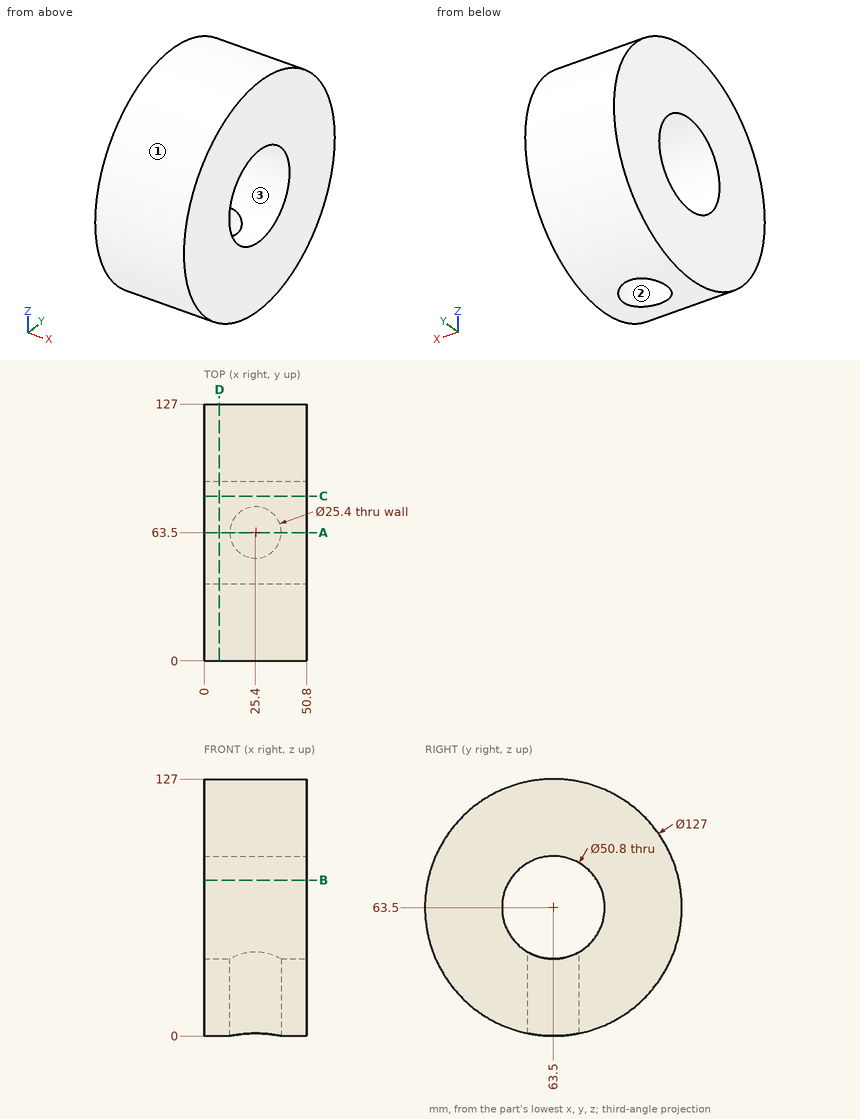
Check sheet for the drawn part. Datum: minimum x, y, z corner. Units: mm. Coordinates: 2 decimals unless noted, no trailing zeros. Loops run counter-clockwise (first coordinate to the right, second up) from the corner with the lowest first, then second, coordinate; pieces in that order, holes last. Notation, with made-up numbers: (-35, 84) -> (-10, 84) arc R5 cw to (-10, 92) -> close; hole circle Ø6 at (57.5, 59.5). An arc over 180 degrees is marked (long way). Answer in a Markdown table with one row per item.
1) Section check B-B (z = 77). Record the cut outline in (x, y).
The answers:
| item | result |
|---|---|
| outline | (0, 1.45) -> (50.8, 1.45) -> (50.8, 41.98) -> (0, 41.98) -> close; (0, 85.02) -> (50.8, 85.02) -> (50.8, 125.55) -> (0, 125.55) -> close |
2) Draft check along Z on the marked faces 1, 2 and 3. Enter one of: released by +Z, released by -Z, zero draft, split by the parting line, or undercut.
The answers:
| item | result |
|---|---|
| face 1 | split by the parting line |
| face 2 | zero draft |
| face 3 | undercut |
3) Depth check by flat-ended pin: P1, Ø15, axis at x = 25.4, y = 63.5, coming from the +Z side; P2, Ø5, axis at x = 34.5, y = 47, coming from the -Z side; P3, Ø10, axis at x = 26.5, y = 77.5, coming from the -Z side. Enter the tip coordinate at first touch or a pass-through.
The answers:
| item | result |
|---|---|
| P1 | stops at z = 127 |
| P2 | stops at z = 1.56 |
| P3 | stops at z = 1.05 |
4) Scan lines: line 1 along X through (y, z) = (63, 25); line 2 along Z through (x, y) = (39, 63); line 3 along Z through (x, y) = (36, 63). Record each from-to range of solid material in increasing order. Write a range as from..to.
The answers:
| item | result |
|---|---|
| line 1 | x = 0..12.71, 38.09..50.8 |
| line 2 | z = 0..38.1, 88.9..127 |
| line 3 | z = 88.9..127 |
5) Section check A-A (y = 63.5). Record the cut outline in (x, z), and give its area (3 significant figures).
The answers:
| item | result |
|---|---|
| outline | (0, 0) -> (12.7, 0) -> (12.7, 38.1) -> (0, 38.1) -> close; (0, 88.9) -> (50.8, 88.9) -> (50.8, 127) -> (0, 127) -> close; (38.1, 0) -> (50.8, 0) -> (50.8, 38.1) -> (38.1, 38.1) -> close |
| area | 2,900 mm2 |
6) Section check C-C (y = 81.5). Record the cut outline in (x, z), and give its area (3 significant figures).
The answers:
| item | result |
|---|---|
| outline | (0, 2.6) -> (50.8, 2.6) -> (50.8, 45.58) -> (0, 45.58) -> close; (0, 81.42) -> (50.8, 81.42) -> (50.8, 124.4) -> (0, 124.4) -> close |
| area | 4,370 mm2 |
7) Section check D-D (x = 7.5). Record the cut outline in (y, z).
The answers:
| item | result |
|---|---|
| outline | circle Ø127 at (63.5, 63.5); hole circle Ø50.8 at (63.5, 63.5) |
